Geometry check sheet. Reference: drawing and pictorial views, mm from the part's lowest x, y, z. A direction names the side the tool comes from. Round coordinates to 2 decimals unless told otherwise and drop trailing zeros. Loops run counter-clockwise (first coordinate to the right, second up) from the corner with the lowest first, then second, coordinate; pieces in that order, holes last. Notation, with made-up numbers: (-31.5, 79.5) - (0.5, 79.5) arc R11 cw to (0.5, 88.5) - close; hole circle Ø9 at (32.25, 31.25). An arc over 180 degrees is marked (long way). Return JSON: item names as keys, results as strings.
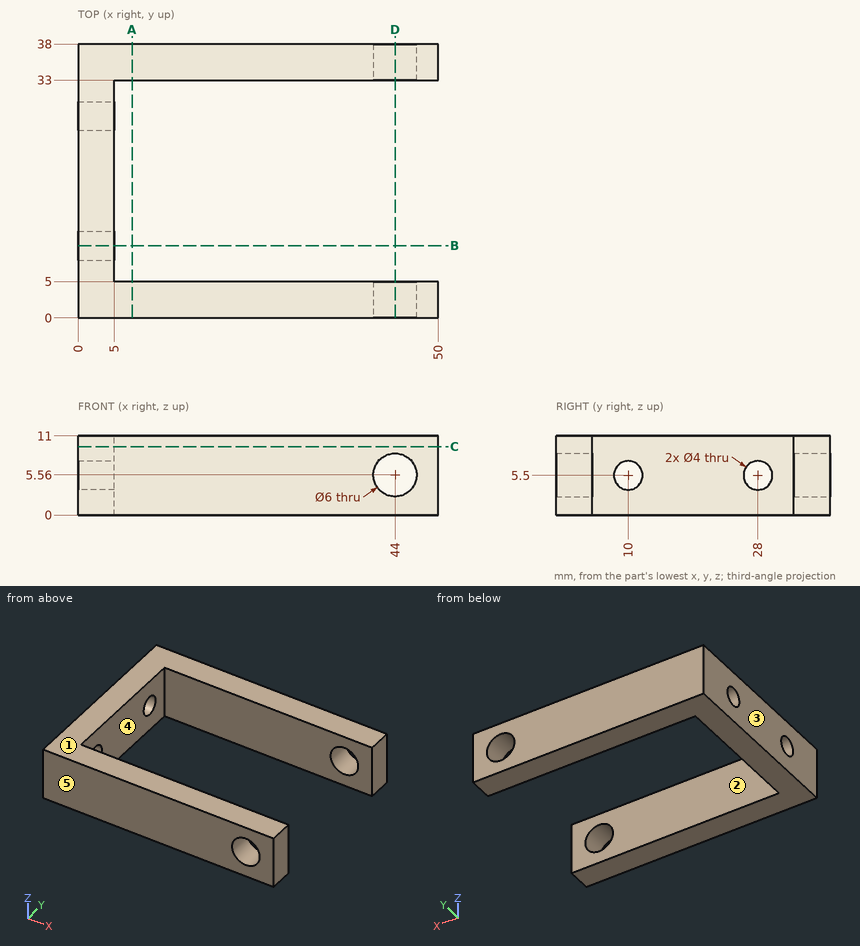
Q1. Tool access check on the marked faces 1 and 2. Record the directions out of +Z, -Z, +X, -X, +Y, -Y that give a thin tool (end or side, any length) a straight path to the whole face; none if there is none.
Answer key:
{"face 1": "+Z, +X, -X, +Y, -Y", "face 2": "+Z, -Z, +X"}
Q2. Sectioned sample at C-C (z = 9.5). Enter the section's corners in (x, y), plus the area to 3 significant figures.
Answer key:
{"outline": "(0, 0) - (50, 0) - (50, 5) - (5, 5) - (5, 33) - (50, 33) - (50, 38) - (0, 38) - close", "area": "640 mm²"}
Q3. Depth check by flat-ended pin: P1, Ø2.5, axis at y = 28, z = 5.5, coming from the -X side; P2, Ø3.5, axis at y = 18.5, z = 4, coming from the +X side. Enter the tip coordinate at first touch or a pass-through.
Answer key:
{"P1": "passes through", "P2": "stops at x = 5"}
Q4. Sectioned sample at D-D (x = 44). Enter the section's corners in (y, z).
Answer key:
{"outline": "(0, 0) - (5, 0) - (5, 2.56) - (0, 2.56) - close; (0, 8.56) - (5, 8.56) - (5, 11) - (0, 11) - close; (33, 0) - (38, 0) - (38, 2.56) - (33, 2.56) - close; (33, 8.56) - (38, 8.56) - (38, 11) - (33, 11) - close"}
Q5. Sectioned sample at A-A (x = 7.5). Enter the section's corners in (y, z).
Answer key:
{"outline": "(0, 0) - (5, 0) - (5, 11) - (0, 11) - close; (33, 0) - (38, 0) - (38, 11) - (33, 11) - close"}
Q6. Sectioned sample at B-B (y = 10). Enter the section's corners in (x, z), plus the area to 3 significant figures.
Answer key:
{"outline": "(0, 0) - (5, 0) - (5, 3.5) - (0, 3.5) - close; (0, 7.5) - (5, 7.5) - (5, 11) - (0, 11) - close", "area": "35.0 mm²"}
Q7. Draft check along Y on the marked faces 3, 4 and 5. Enter one of: released by +Y, released by -Y, zero draft, split by the parting line, or undercut.
Answer key:
{"face 3": "zero draft", "face 4": "undercut", "face 5": "released by -Y"}
Q8. Scan lines: probe 1 along Y at (x, z) = (3.7, 5.5); probe 2 along Y at (x, z) = (26, 7.25); probe 3 along X at (y, z) = (18, 4). Record each from-to range of solid material in increasing order. Write a range as [from, to].
Answer key:
{"probe 1": "y = [0, 8], [12, 26], [30, 38]", "probe 2": "y = [0, 5], [33, 38]", "probe 3": "x = [0, 5]"}
